Here's how the part is built. I have some questions about the finished solid (model axes, mm). Face numbers are marked on the shaded views. Give positions to 0.01 mm unless a question says otherwise; leave off trailing zeros. Use CSV: the item, a comma, the result in double quotes. Start each with the question number.
(1) For pin 1 Ø2 at (y, z) = (2, 8.5) entering from +X; pin 2 Ø1.5 at (x, y) = (4, 7.5) entering from +Z; pin 3 Ø3 at (y, z) = (7.5, 6) entering from -X; pin 4 Ø6 at (x, y) = (1.5, 5.5) entering from -Z (3 decimals), each with a flat end and sliding along its axis, tell me the tip position at first contact or that it passes through.
(2) If we mould it in two halves opening along Y, with no side actions, what happens to the marked faces 1, 2 and 3? For each: pulls with the +Y half, pulls with the -Y half, needs draft (parallel to the pull), parting line crosses it, or undercut.
(3) I need wall thicknesses on L1, parallel to Y at x = 8.5, z = 6.75; L2, parallel to Y at x = 8.25, z = 5.75; L3, parallel to X at y = 1.5, z = 6.75. Which ranges of each line are inside material? Lowest first, please. Write a range as [from, to].
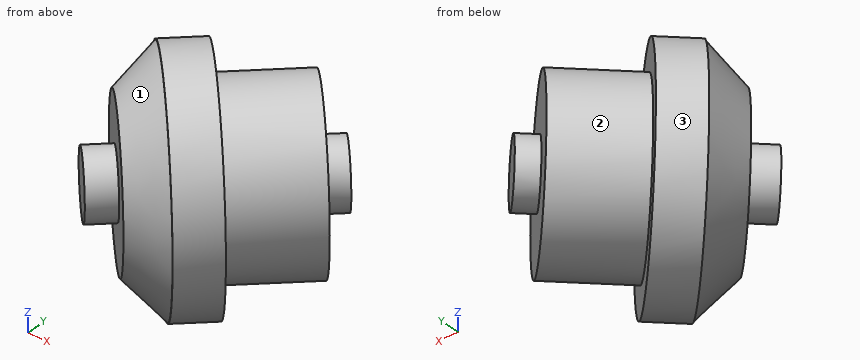
from build123d import *

# Parameters (mm, degrees)
CYLINDER081016_R                               = 1.5
CYLINDER081016_DEPTH                           = 10
CYLINDER081017_R                               = 4
CYLINDER081017_DEPTH                           = 4
CYLINDER081018_R                               = 5.355
CYLINDER081018_DEPTH                           = 2
FUSION103077013004017008011030_PLACEMENT_ANGLE = 45


with BuildPart() as cylinder081013:
    # Cylinder081016 → Cylinder081016 (new body)
    with BuildSketch(Plane(origin=(0, 12, 8), x_dir=(1, 0, 0), z_dir=(0, -1, 0))):
        Circle(CYLINDER081016_R)
    extrude(amount=CYLINDER081016_DEPTH)


with BuildPart() as cylinder081014:
    # Cylinder081017 → Cylinder081017 (new body)
    with BuildSketch(Plane(origin=(0, 11, 8), x_dir=(1, 0, 0), z_dir=(0, -1, 0))):
        Circle(CYLINDER081017_R)
    extrude(amount=CYLINDER081017_DEPTH)


with BuildPart() as cylinder081015:
    # Cylinder081018 → Cylinder081018 (new body)
    with BuildSketch(Plane(origin=(0, 7, 8), x_dir=(1, 0, 0), z_dir=(0, -1, 0))):
        Circle(CYLINDER081018_R)
    extrude(amount=CYLINDER081018_DEPTH)


with BuildPart() as commercial_gear:
    # Cone004 → Cone004 (revolve)
    with BuildSketch(Plane(origin=(0, 5, 8), x_dir=(1, 0, 0), z_dir=(0, 0, -1))):
        Polygon((0, 0), (5.31, 0), (3.6, 1.71), (0, 1.71), align=None)
    revolve(axis=Axis((0, 5, 8), (0, -1, 0)))

    # Fusion103077013004017008011030: union Cylinder081013, Cylinder081014, Cylinder081015
    add(cylinder081013.part)
    add(cylinder081014.part)
    add(cylinder081015.part)


with BuildPart() as commercial_gear_1:
    # Fusion103077013004017008011030 placement: moved
    add(commercial_gear.part.rotate(Axis((0, 0, 0), (0, 0, -1)), FUSION103077013004017008011030_PLACEMENT_ANGLE))


solid = commercial_gear_1.part
Geometry says:
1,pin 1,"x = 8.74"
1,pin 2,"z = 11.61"
1,pin 3,"x = -0.23"
1,pin 4,"z = 2.645"
2,face 1,"pulls with the -Y half"
2,face 2,"undercut"
2,face 3,"parting line crosses it"
3,L1,"[1.14, 1.4], [3.13, 7.06], [7.33, 8.47]"
3,L2,"[1.38, 1.65], [3.57, 7.31]"
3,L3,"[1.33, 2.67], [3.15, 8.4]"
